```python
from build123d import *

# Parameters (mm, degrees)
F1_DEPTH    = 8
F2_T4_DEPTH = 33.981320863
F3_T4_DEPTH = 33.981320863
F4_R        = 3.99999
F5_R        = 1.75
F6_DEPTH    = 10
F7_R        = 1.75
F8_DEPTH    = 10


# Not quite as in the source:
# - a fillet or chamfer that OpenCascade refuses, or shapes differently, is made with other operations: its cross-section is extruded or revolved along the edge and cut away or added
# - a fillet or chamfer is up to 0.001 mm smaller than in the source, because OpenCascade refuses the exact size


with BuildPart() as f1:
    # F0 (on Front) → F1 (new body)
    with BuildSketch(Plane.XZ):
        Polygon((14, 65.5), (10, 65.5), (10, 63.5), (12, 63.5), (12, 61.5), (16.5, 61.5), (16.5, 58.5), (16.5, 53.5), (14.5, 53.5), (14.5, 58.5), (10, 58.5), (10, 55.5), (11.5, 55.5), (11.5, 51.5), (18.5, 51.5), (18.5, 63.5), (14, 63.5), align=None)
        Polygon((10, 11.5), (10, 9.5), (14, 9.5), (14, 11.5), (18.5, 11.5), (18.5, 23.5), (11.5, 23.5), (11.5, 19.5), (10, 19.5), (10, 16.5), (14.5, 16.5), (14.5, 21.5), (16.5, 21.5), (16.5, 16.5), (16.5, 13.5), (12, 13.5), (12, 11.5), align=None)
        Polygon((0, 75), (0, 0), (10, 0), (10, 7.5), (3, 7.5), (3, 9.5), (3, 13.5), (3, 16.5), (3, 17.5), (5, 17.5), (5, 16.5), (10, 16.5), (10, 19.5), (3, 19.5), (3, 21.5), (10, 21.5), (10, 53.5), (3, 53.5), (3, 55.5), (10, 55.5), (10, 58.5), (5, 58.5), (5, 57.5), (3, 57.5), (3, 58.5), (3, 61.5), (3, 65.5), (3, 67.5), (10, 67.5), (10, 75), align=None)
    extrude(amount=F1_DEPTH)

    # F2: chamfer of 1 x 5 on 1 edges, made by hand


with BuildPart() as f2_tool2:
    # F2_s3 → F2_t4 (new body)
    with BuildSketch(Plane.XZ.offset(-12.9906604315)):
        Polygon((11.5, 56.5), (12.5, 51.5), (11.5, 51.5), align=None)
    extrude(amount=F2_T4_DEPTH)

    split(bisect_by=Plane.XY.offset(55.5), keep=Keep.BOTTOM)


with BuildPart() as f1_1:
    add(f1.part)

    # F2_t1: cut F2_tool2
    add(f2_tool2.part, mode=Mode.SUBTRACT)

    # F3: chamfer of 5 x 1 on 1 edges, made by hand


with BuildPart() as f3_tool2:
    # F3_s3 → F3_t4 (new body)
    with BuildSketch(Plane.XZ.offset(-12.9906604315)):
        Polygon((11.5, 18.5), (12.5, 23.5), (11.5, 23.5), align=None)
    extrude(amount=F3_T4_DEPTH)

    split(bisect_by=Plane.XY.offset(19.5), keep=Keep.TOP)


with BuildPart() as f1_2:
    add(f1_1.part)

    # F3_t1: cut F3_tool2
    add(f3_tool2.part, mode=Mode.SUBTRACT)

    # F4 (radius 4 in the source; OpenCascade refuses exactly that, so slightly less here)
    f4_edges = [f1_2.edges().sort_by_distance(p)[0] for p in [
        (5, -8, 75),
        (5, 0, 75),
        (5, -8, 0),
        (5, 0, 0),
    ]]
    fillet(f4_edges, radius=F4_R)

    # F5 (on face) → F6 (cut)
    with BuildSketch(Plane.YZ.offset(10)):
        with Locations((-4, 71)):
            Circle(F5_R)
    extrude(amount=-F6_DEPTH, mode=Mode.SUBTRACT)

    # F7 (on face) → F8 (cut)
    with BuildSketch(Plane.YZ.offset(10)):
        with Locations((-4, 4)):
            Circle(F7_R)
    extrude(amount=-F8_DEPTH, mode=Mode.SUBTRACT)


solid = f1_2.part
```
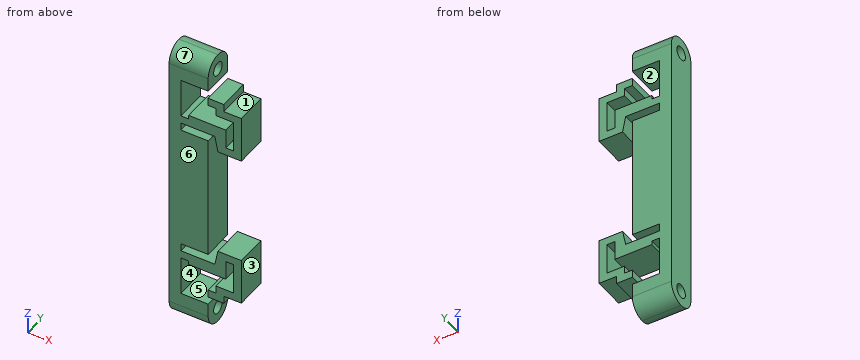
The model under review builds one solid part; all positions refer to its coordinate system, in mm. Face numbers are marked on the shaded views. A direction names the side the tool comes from. Coordinates: 2 decimals unless noted, no trailing zeros. Write each loop counter-clockwise with the first axis right and the second up, starting at its lowest first coordinate (ties: lowest second). Pieces come first, ordered by that corner, then holes. Notation, with made-up numbers: (-39, 21) - (-14, 21) arc R11 ccw to (-14, 37) - close; hole circle Ø4 at (-37.75, 26). An arc over 180 degrees is marked (long way). Answer in a Markdown table with one row per item. Add a question column.
Q1. Draft analysis for pull direction Z (two halves, no side actions). For the marked faces 5, 6 and 7, state which applies: +Z half, -Z half, draft (parallel to the pull), parting line (faces both ways), or undercut.
Q2. Consider section B-B on x = 17.25. Give the boundary of the cut face in (y, z), then the cut area to 3 significant figures.
Q3. For the marked faces 1, 2, 3 and 4, list the 3-axis set-ups (+Z, -Z, +X, -X, +Y, -Y) from which the entire face can be reached by the end or side of a thin tool; tool diameter is ignored.
Q4. Clearance check with flat-ended pins moving along their axes: pin 1 (2 mm diameter, centred on x = 15.5, y = -4, fed in from -Z); pin 2 (1 mm diameter, centred on y = -2.5, z = 10, fed in from +X); pin 3 (2 mm diameter, centred on x = 7, y = -2.5, fed in from -Z). State where each tip first meets the part, or that it passes through.
Q5. To check wall thickness, follow line 1 along Z through (x, y) = (10.25, -5.5); line 2 along Z through (x, y) = (17.5, -4.5); line 3 along Y through (x, z) = (4, 71). State the ranges of each line that lie inside material, in increasing order. Write a range as from..to.
Q6. Consider section A-A on x = 6. Give the number of separate pieces and of enclosed holes in the cut face, then the cut area to 3 significant figures.
Q7. Consider section C-C on z = 40.5. Give the boundary of the cut face in (x, y), then the cut area to 3 significant figures.
Answers below:
| question | item | result |
|---|---|---|
| 1 | face 5 | undercut |
| 1 | face 6 | draft |
| 1 | face 7 | +Z half |
| 2 | outline | (-8, 11.5) - (0, 11.5) - (0, 23.5) - (-8, 23.5) - close; (-8, 51.5) - (0, 51.5) - (0, 63.5) - (-8, 63.5) - close |
| 2 | area | 192 mm² |
| 3 | face 1 | +Z, +X, +Y, -Y |
| 3 | face 2 | +X, +Y, -Y |
| 3 | face 3 | +Z, -Z, +X, +Y, -Y |
| 3 | face 4 | +Y, -Y |
| 4 | pin 1 | z = 11.5 |
| 4 | pin 2 | x = 14 |
| 4 | pin 3 | z = 0.03 |
| 5 | line 1 | 9.5..11.5, 16.5..19.5, 55.5..58.5, 63.5..65.5 |
| 5 | line 2 | 11.5..23.5, 51.5..63.5 |
| 5 | line 3 | -8..-5.75, -2.25..0 |
| 6 | separate pieces | 5 |
| 6 | enclosed holes | 2 |
| 6 | area | 391 mm² |
| 7 | outline | (0, -8) - (10, -8) - (10, 0) - (0, 0) - close |
| 7 | area | 80.0 mm² |
